from build123d import *

# Parameters (mm, degrees)
BOSS_EXTRU_1_DEPTH           = 20
ESQUISSE3_R                  = 5
ENL_V_MAT_EXTRU_1_DEPTH      = 20
CONG_1_R                     = 10
ENL_V_MAT_EXTRU_3_DEPTH      = 42.231056256
ENL_V_MAT_EXTRU_3_DEPTH_BACK = 42.231056256
ESQUISSE1_4_R                = 2
ESQUISSE1_5_R                = 4
ENL_V_MAT_EXTRU_4_DEPTH      = 2
ENL_V_START                  = 18
ESQUISSE1_6_R                = 4
ENL_V_MAT_EXTRU_5_DEPTH      = 2
BOSS_EXTRU_4_DEPTH           = 20
BOSS_EXTRU_5_START           = 5
BOSS_EXTRU_5_DEPTH           = 5
CONG_3_START                 = -24
CONG_3_DEPTH                 = 7.5
CONG_4_START                 = 16.9999999
CONG_4_DEPTH                 = 4.0000001
ENL_V_MAT_EXTRU_6_DEPTH      = 2
ENL_V_MAT_EXTRU_6_DEPTH_BACK = 43.500000171
ESQUISSE7_R                  = 5.1
BOSS_EXTRU_7_START           = 2
ESQUISSE9_R                  = 10
ESQUISSE9_R_2                = 5.1
BOSS_EXTRU_7_DEPTH           = 2


with BuildPart() as part:
    # Esquisse1 → Boss.-Extru.1 (new body)
    with BuildSketch(Plane.XY):
        with BuildLine():
            Line((0, 20), (-30, 20))
            Line((-30, 20), (-30, -20))
            Line((-30, -20), (0, -20))
            ThreePointArc((0, -20), (20, 0), (0, 20))
        make_face()
    extrude(amount=BOSS_EXTRU_1_DEPTH)

    # Esquisse3 → Enlèv. mat.-Extru.1 (cut)
    with BuildSketch(Plane.ZY.offset(30)):
        with Locations(Location((10, 0, 0), (0, 0, 270))):
            Circle(ESQUISSE3_R)
    extrude(amount=-ENL_V_MAT_EXTRU_1_DEPTH, mode=Mode.SUBTRACT)

    # Congé1
    cong_1_edges = [part.edges().sort_by_distance(p)[0] for p in [
        (-30, 20, 10),
        (-30, -20, 10),
    ]]
    fillet(cong_1_edges, radius=CONG_1_R)

    # Esquisse1<4> → Enlèv. mat.-Extru.3 (cut, two sides: drawn at the far end of the back side and taken through both)
    with BuildSketch(Plane.XY.offset(-ENL_V_MAT_EXTRU_3_DEPTH_BACK)):
        with Locations((-23.5, 0)):
            Circle(ESQUISSE1_4_R)
    extrude(amount=ENL_V_MAT_EXTRU_3_DEPTH + ENL_V_MAT_EXTRU_3_DEPTH_BACK, mode=Mode.SUBTRACT)

    # Esquisse1<5> → Enlèv. mat.-Extru.4 (cut)
    with BuildSketch(Plane.XY):
        with Locations((-23.5, 0)):
            Circle(ESQUISSE1_5_R)
    extrude(amount=ENL_V_MAT_EXTRU_4_DEPTH, mode=Mode.SUBTRACT)

    # Esquisse1<6> → Enlèv. mat.-Extru.5 (cut)
    with BuildSketch(Plane.XY.offset(ENL_V_START)):
        with Locations((-23.5, 0)):
            Circle(ESQUISSE1_6_R)
    extrude(amount=ENL_V_MAT_EXTRU_5_DEPTH, mode=Mode.SUBTRACT)

    # Esquisse5 → Boss.-Extru.4 (add)
    with BuildSketch(Plane.XY.offset(20)):
        with BuildLine():
            Line((20, 0), (20, -16.5))
            ThreePointArc((20, -16.5), (18.242640687, -20.742640687), (14, -22.5))
            Line((14, -22.5), (-24, -22.5))
            ThreePointArc((-24, -22.5), (-28.242640687, -20.742640687), (-30, -16.5))
            Line((-30, -16.5), (-30, -10))
            ThreePointArc((-30, -10), (-27.071067812, -17.071067812), (-20, -20))
            Line((-20, -20), (0, -20))
            ThreePointArc((0, -20), (14.142135624, -14.142135624), (20, 0))
        make_face()
    extrude(amount=-BOSS_EXTRU_4_DEPTH)

    # Esquisse6 → Boss.-Extru.5 (add)
    with BuildSketch(Plane.XY.offset(20).offset(BOSS_EXTRU_5_START)):
        with BuildLine():
            Line((20, -16.5), (18.5, -16.5))
            ThreePointArc((18.5, -16.5), (17.181980515, -19.681980515), (14, -21))
            Line((14, -21), (14, -22.5))
            ThreePointArc((14, -22.5), (18.242640687, -20.742640687), (20, -16.5))
        make_face()
    extrude(amount=-BOSS_EXTRU_5_DEPTH)

    # Congé3: read off the stored shape, not the designer's step
    # Congé3 outline → Congé3 (cut)
    with BuildSketch(Plane(origin=(0, 0, 0), x_dir=(1, 0, 0), z_dir=(0, 1, 0)).offset(CONG_3_START)):
        with BuildLine():
            Line((14, -25), (17, -25))
            add(Edge.make_bspline(
                [(17, -25), (14, -25), (14, -22)],
                knots=[0, 0, 0, 1, 1, 1], degree=2, weights=[1, 0.707106781, 1]))
            Line((14, -22), (14, -25))
        make_face()
    extrude(amount=CONG_3_DEPTH, mode=Mode.SUBTRACT)

    # Congé4: read off the stored shape, not the designer's step
    # Congé4 outline → Congé4 (cut)
    with BuildSketch(Plane.YZ.offset(CONG_4_START)):
        with BuildLine():
            Line((-16.5, 25), (-19.5, 25))
            add(Edge.make_bspline(
                [(-19.5, 25), (-16.5, 25), (-16.5, 22)],
                knots=[0, 0, 0, 1, 1, 1], degree=2, weights=[1, 0.707106781, 1]))
            Line((-16.5, 22), (-16.5, 25))
        make_face()
    extrude(amount=CONG_4_DEPTH, mode=Mode.SUBTRACT)

    # Esquisse7 → Enlèv. mat.-Extru.6 (cut, two sides: drawn at the far end of the back side and taken through both)
    with BuildSketch(Plane.XY.offset(20).offset(-ENL_V_MAT_EXTRU_6_DEPTH_BACK)):
        Circle(ESQUISSE7_R)
    extrude(amount=ENL_V_MAT_EXTRU_6_DEPTH + ENL_V_MAT_EXTRU_6_DEPTH_BACK, mode=Mode.SUBTRACT)

    # Esquisse9 → Boss.-Extru.7 (add)
    with BuildSketch(Plane.XY.offset(20).offset(BOSS_EXTRU_7_START)):
        Circle(ESQUISSE9_R)
        Circle(ESQUISSE9_R_2, mode=Mode.SUBTRACT)
    extrude(amount=-BOSS_EXTRU_7_DEPTH)


solid = part.part
Model file for the job. Use its own axes, mm. A direction names the side the tool comes from. Round coordinates to 2 decimals unless told otherwise and drop trailing zeros. Order: outer loops, then holes, each group sorted by start corner. A loop starts at its lowest first (then second) coordinate and runs counter-clockwise, first axis right, second up. Notation, with made-up numbers: M 48.5,85 L 84.5,85 A27 cw 84.5,113 Z; hole C 39,-29 d11. An arc over 180 degrees is marked long. Write each question's results on one line, items separated by ' | '. Start each with the question number.
(1) Probe probe 1 along Z at (x, y) = (1, 7); probe 2 along Z at (x, y) = (5.5, 12); probe 3 along Y at (x, z) = (-4, 4). List the from-to ranges inside material, lowest first. Write a range as from..to.
(2) Two-plate mould, pull along Z, no slides. Class faces 1 (the face through (-20.14, -4.77, 11.5)), 2 (the face through (-22, -2, 2)), 3 (the face through (-21.592, 0.601, 16.267)): pulls with the +Z half, pulls with the -Z half, needs draft (parallel to the pull), parting line crosses it, or undercut.
(3) Saw through at D-D, the plane z = 12.25. Give the cut face in (x, y), then the cut area to 3 significant figures.
(4) Drop flat-ended pins along their axis: pin 1 (4 mm diameter, centred on x = -23, y = 4, fed in from +Z); pin 2 (5 mm diameter, centred on x = -23.5, y = 0, fed in from +Z); pin 3 (1.2 mm diameter, centred on y = -21.5, z = 21, fed in from -X); pin 4 (16.5 mm diameter, centred on x = 0, y = 0, fed in from -Z). Give the stop position or say it passes through.
(5) Which spindle directions (+Z, -Z, +X, -X, +Y, -Y) get a long thin tool onto all of the face, cutting with end or side? Do faces 4 (the face through (14, -22, 21)), 5 (the face through (-26.7, -2.4, 19)), 6 (the face through (19, -16.5, 21)), 7 (the face through (17.217, -19.647, 22.535)). Say none if no direction does.
(6) Saw through at B-B, the plane x = 1.5. Give the cut face in (y, z).
(7) Saw through at A-A, the plane z = 16. Give the cut face in (x, y), then the cut area to 3 significant figures.
(8) Saw through at C-C, the plane z = 8.5. Give the cut face in (x, y), then the cut area to 3 significant figures.
Established:
1) probe 1: z = 0..22 | probe 2: z = 0..20 | probe 3: y = -22.5..-3.16, 3.16..20
2) face 1: undercut | face 2: pulls with the -Z half | face 3: needs draft
3) outline: M -30,-16.5 A6 ccw -24,-22.5 L 14,-22.5 A6 ccw 20,-16.5 L 20,0 A20 ccw 0,20 L -20,20 A10 ccw -30,10 L -30,4.47 L -10,4.47 L -10,-4.47 L -30,-4.47 Z; hole C 0,0 d10.2 | area: 1,740 mm^2
4) pin 1: stops at z = 20 | pin 2: stops at z = 18 | pin 3: stops at x = 14 | pin 4: stops at z = 0
5) face 4: +Z, -X, +Y, -Y | face 5: +Z | face 6: +Z, +X, -X, +Y | face 7: +Z, -X, +Y
6) outline: M -22.5,0 L -4.87,0 L -4.87,22 L -9.89,22 L -9.89,20 L -22.5,20 Z; M 4.87,0 L 19.94,0 L 19.94,20 L 9.89,20 L 9.89,22 L 4.87,22 Z
7) outline: M -30,-16.5 A6 ccw -24,-22.5 L 14,-22.5 A6 ccw 20,-16.5 L 20,0 A20 ccw 0,20 L -20,20 A10 ccw -30,10 Z; hole C -23.5,0 d4; hole C 0,0 d10.2 | area: 1,910 mm^2
8) outline: M -30,-16.5 A6 ccw -24,-22.5 L 14,-22.5 A6 ccw 20,-16.5 L 20,0 A20 ccw 0,20 L -20,20 A10 ccw -30,10 L -30,4.77 L -10,4.77 L -10,-4.77 L -30,-4.77 Z; hole C 0,0 d10.2 | area: 1,730 mm^2
